Build history of the part. All positions in model axes, mm. Coordinates: 2 decimals unless noted, no trailing zeros. Order: outer loops, then holes, each group sorted by start corner. A loop starts at its lowest first (then second) coordinate and runs counter-clockwise, first axis right, second up. Notation, with made-up numbers: (55.25, 28.5) - (112.25, 28.5) arc R14 cw to (112.25, 53.5) - close; hole circle Ø5 at (68.25, 30). An arc over 180 degrees is marked (long way). Return JSON: item names as keys, results as strings.
from build123d import *

# Parameters (mm, degrees)
BODY_DEPTH           = 4
M5_CLEARANCE_HOLE2_D = 5.5


with BuildPart() as part:
    # Sketch1 → Body (new body)
    with BuildSketch(Plane(origin=(0, 0, 0), x_dir=(1, 0, 0), z_dir=(0, 1, 0))):
        Polygon((0, 4.618802154), (-4, 2.309401077), (-4, -2.309401077), (0, -4.618802154), (4, -2.309401077), (4, 2.309401077), align=None)
    extrude(amount=BODY_DEPTH)

    # Sketch5 → Loft1 section 0
    with BuildSketch(Plane(origin=(0, 4, 0), x_dir=(1, 0, 0), z_dir=(0, 1, 0))):
        with BuildLine():
            Line((3.75, 2.165063509), (0, 4.330127019))
            Line((0, 4.330127019), (-3.75, 2.165063509))
            Line((-3.75, 2.165063509), (-3.75, -2.165063509))
            Line((-3.75, -2.165063509), (0, -4.330127019))
            Line((0, -4.330127019), (3.75, -2.165063509))
            Line((3.75, -2.165063509), (3.75, 2.165063509))
        make_face()
    # Sketch4 for Loft1 → Loft1 section 1
    with BuildSketch(Plane(origin=(0, 5, 0), x_dir=(1, 0, 0), z_dir=(0, 1, 0))):
        with BuildLine():
            # circular arc as an exact rational Bezier (weights 1, cos(half-angle), 1)
            Bezier((3.031088913, 1.75), (2.020725942, 3.5), (0, 3.5), weights=[1, 0.866025404, 1])
            Bezier((0, 3.5), (-2.020725942, 3.5), (-3.031088913, 1.75), weights=[1, 0.866025404, 1])
            Bezier((-3.031088913, 1.75), (-4.041451885, 0), (-3.031088913, -1.75), weights=[1, 0.866025404, 1])
            Bezier((-3.031088913, -1.75), (-2.020725942, -3.5), (0, -3.5), weights=[1, 0.866025404, 1])
            Bezier((0, -3.5), (2.020725942, -3.5), (3.031088913, -1.75), weights=[1, 0.866025404, 1])
            Bezier((3.031088913, -1.75), (4.041451885, 0), (3.031088913, 1.75), weights=[1, 0.866025404, 1])
        make_face()
    loft()

    # M5 Clearance Hole2 (through all)
    with Locations(Plane(origin=(0, 5, 0), x_dir=(1, 0, 0), z_dir=(0, 1, 0))):
        with Locations((0, 0)):
            Hole(M5_CLEARANCE_HOLE2_D / 2)


solid = part.part
1. Drop flat-ended pins along their axis: pin 1 (1 mm diameter, centred on y = 1.5, z = -3, fed in from +X); pin 2 (2.5 mm diameter, centred on x = -0.5, z = 1.5, fed in from +Y); pin 3 (2 mm diameter, centred on x = -1, y = 4.5, fed in from -Z). Give the stop position or say it passes through.
Check values:
{"pin 1": "x = 3.67", "pin 2": "y = 5", "pin 3": "z = -4.54"}
2. Probe L1, parallel to Z at x = -0.5, y = 3.1; L2, parallel to Z at x = -2.25, y = 3.4; L3, parallel to X at y = 3.25, z = 1.75. List the from-to ranges inside material, lowest first.
Check values:
{"L1": "-4.33 to -2.7, 2.7 to 4.33", "L2": "-3.32 to -1.58, 1.58 to 3.32", "L3": "-4 to -2.12, 2.12 to 4"}
3. Mould opens along Z. For faces 1 (the cylindrical face through (0.596, 2.465, 2.685)), 2 (the flat face through (1.97, 1.97, 3.48)), 3 (the flat face through (2.028, 1.972, -3.448)) say: pulls with the +Z half, pulls with the -Z half, needs draft (parallel to the pull), parting line crosses it, or undercut.
Check values:
{"face 1": "undercut", "face 2": "pulls with the +Z half", "face 3": "pulls with the -Z half"}
4. Cut at A-A on y = 1.6. Give the cut face in (x, z).
Check values:
{"outline": "(-4, -2.31) - (0, -4.62) - (4, -2.31) - (4, 2.31) - (0, 4.62) - (-4, 2.31) - close; hole circle Ø5.5 at (0, 0)"}
